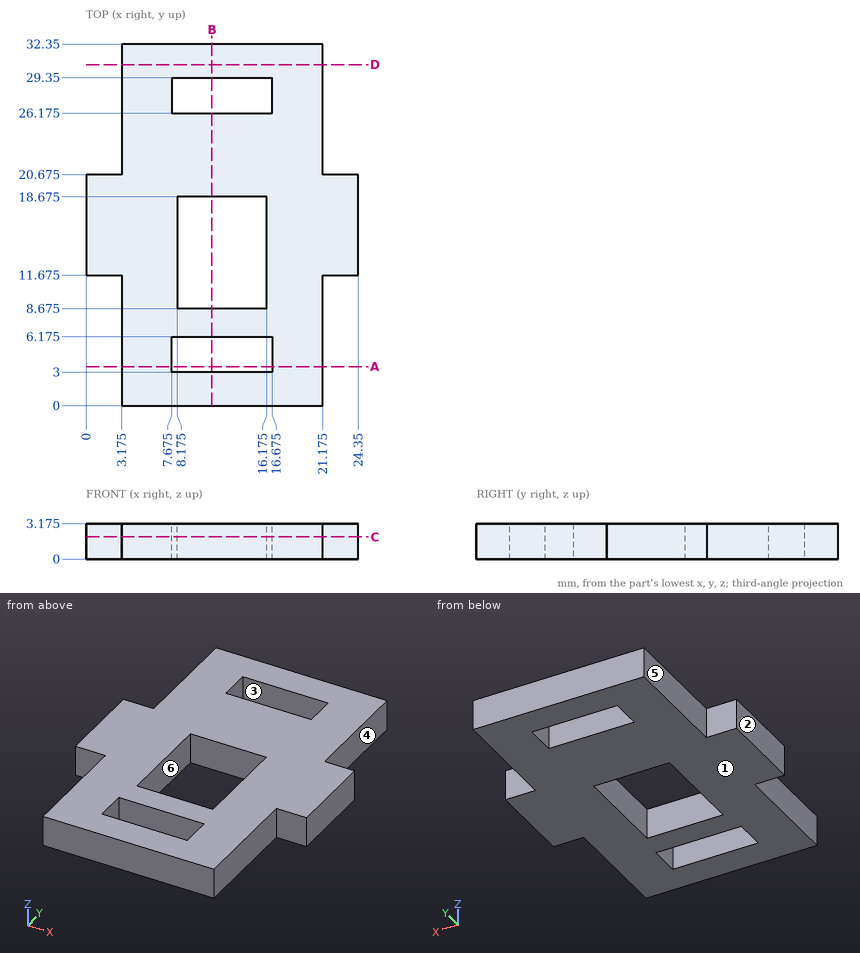
Geometry: see drawing. Coordinates: mm, zero at the bounding-box minimum. A direction names the side the tool comes from. Give positions to 0.01 mm unless a question says otherwise; leave off trailing zeros. Write each loop counter-clockwise with the first axis right and the second up, starting at its lowest first coordinate (ties: lowest second). Pieces come first, ordered by that corner, then holes. Notation, with made-up numbers: M -37.5,58.5 L 18.5,58.5 A4 ccw 18.5,65.5 Z; hole C -13.75,55 d6. An arc over 180 degrees is marked long. Return JSON: item names as keys, results as strings. Group by question number.
1) Cut plane A-A, the plane y = 3.5. Output: boundary loops of the cut face in (x, z) (3 decimals).
2) First-contact query: pin 1 Ø5 at (x, y) = (10, 3.5) entering from +Z (3 decimals); pin 2 Ø1 at (y, z) = (4, 1.5) entering from -X (3 decimals); pin 3 Ø1.6 at (x, z) = (1, 2) entering from +Y (3 decimals); pin 4 Ø1.6 at (y, z) = (4.5, 1) entering from +X (3 decimals). Flat tips, straight axial feed; report the tip coordinate or a pass-through.
3) Draft query along X for the marked faces 1, 2 and 3. Return one class per face: released by +X, released by -X, zero draft, split by the parting line, or undercut.
4) Cut plane B-B, the plane x = 11.25. Output: boundary loops of the cut face in (y, z) (3 decimals).
5) Cut plane D-D, the plane y = 30.5. Output: boundary loops of the cut face in (x, z) (3 decimals), then the cut area to 4 significant figures.
6) Cut plane C-C, the plane z = 2. Output: boundary loops of the cut face in (x, y) (3 decimals).
7) Set-up query: the marked faces 4, 5 and 6. Return all of +Z, -Z, +X, -X, +Y, -Y with unobstructed straight access to the full face (end or side cutting, diameter ignored); none if empty.
8) Ray query, L1, parallel to Y at x = 14, z = 1.3 (3 decimals); L2, parallel to X at y = 15.5, z = 2 (3 decimals); L3, parallel to X at y = 11.5, z = 1.8 (3 decimals). Return the intervals inside material, ascending.
Data:
{
 "1": {"outline": "M 3.175,0 L 7.675,0 L 7.675,3.175 L 3.175,3.175 Z; M 16.675,0 L 21.175,0 L 21.175,3.175 L 16.675,3.175 Z"},
 "2": {"pin 1": "stops at z = 3.175", "pin 2": "stops at x = 3.175", "pin 3": "stops at y = 20.675", "pin 4": "stops at x = 21.175"},
 "3": {"face 1": "zero draft", "face 2": "released by -X", "face 3": "undercut"},
 "4": {"outline": "M 0,0 L 3,0 L 3,3.175 L 0,3.175 Z; M 6.175,0 L 8.675,0 L 8.675,3.175 L 6.175,3.175 Z; M 18.675,0 L 26.175,0 L 26.175,3.175 L 18.675,3.175 Z; M 29.35,0 L 32.35,0 L 32.35,3.175 L 29.35,3.175 Z"},
 "5": {"outline": "M 3.175,0 L 21.175,0 L 21.175,3.175 L 3.175,3.175 Z", "area": "57.15 mm²"},
 "6": {"outline": "M 0,11.675 L 3.175,11.675 L 3.175,0 L 21.175,0 L 21.175,11.675 L 24.35,11.675 L 24.35,20.675 L 21.175,20.675 L 21.175,32.35 L 3.175,32.35 L 3.175,20.675 L 0,20.675 Z; hole M 7.675,3 L 16.675,3 L 16.675,6.175 L 7.675,6.175 Z; hole M 7.675,26.175 L 16.675,26.175 L 16.675,29.35 L 7.675,29.35 Z; hole M 8.175,8.675 L 16.175,8.675 L 16.175,18.675 L 8.175,18.675 Z"},
 "7": {"face 4": "+Z, -Z, +X, +Y", "face 5": "+Z, -Z, -X, +Y", "face 6": "+Z, -Z"},
 "8": {"L1": "y = 0 to 3, 6.175 to 8.675, 18.675 to 26.175, 29.35 to 32.35", "L2": "x = 0 to 8.175, 16.175 to 24.35", "L3": "x = 3.175 to 8.175, 16.175 to 21.175"}
}
